Can you work these out from the model? Positions are in its coordinate system, mm. A direction names the side the tool comes from. Round coordinates to 2 decimals unless told otherwise and drop trailing zeros. Order: outer loops, then holes, each group sorted by start corner. A loop starts at its lowest first (then second) coordinate and runs counter-clockwise, first axis right, second up.
from build123d import *

# Parameters (mm, degrees)
SKETCH1_W             = 180
SKETCH1_H             = 75
BOSS_EXTRUDE1_DEPTH   = 3
SKETCH2_W             = 180
SKETCH2_H             = 4
BOSS_EXTRUDE2_DEPTH   = 17
SKETCH3_R             = 1.5
BOSS_EXTRUDE3_DEPTH   = 3
SKETCH4_R             = 0.6
CUT_EXTRUDE1_DEPTH    = 5
SKETCH5_W             = 50
SKETCH5_H             = 33
CUT_EXTRUDE2_DEPTH    = 5
F_3_0MM_DOWEL_HOLE1_D = 3
CUT_EXTRUDE3_REACH    = 100.971
SKETCH8_R             = 1.5
CUT_EXTRUDE4_REACH    = 118.366
SKETCH9_R             = 2.5


with BuildPart() as part:
    # Sketch1 → Boss-Extrude1 (new body)
    with BuildSketch(Plane(origin=(0, 0, 0), x_dir=(1, 0, 0), z_dir=(0, 1, 0))):
        Rectangle(SKETCH1_W, SKETCH1_H)
    extrude(amount=BOSS_EXTRUDE1_DEPTH)

    # Sketch2 → Boss-Extrude2 (add)
    with BuildSketch(Plane(origin=(0, 3, 0), x_dir=(1, 0, 0), z_dir=(0, 1, 0))):
        with Locations((0, 35.5)):
            Rectangle(SKETCH2_W, SKETCH2_H)
    extrude(amount=BOSS_EXTRUDE2_DEPTH)

    # Sketch3 → Boss-Extrude3 (add)
    with BuildSketch(Plane(origin=(0, 3, 0), x_dir=(1, 0, 0), z_dir=(0, 1, 0))):
        with Locations(Location((-80, 29.5, 0), (0, 0, 270))):
            Circle(SKETCH3_R)
        with Locations(Location((-55, 29.5, 0), (0, 0, 270))):
            Circle(SKETCH3_R)
        with Locations(Location((-55, -35.5, 0), (0, 0, 270))):
            Circle(SKETCH3_R)
        with Locations(Location((-80, -35.5, 0), (0, 0, 270))):
            Circle(SKETCH3_R)
    extrude(amount=BOSS_EXTRUDE3_DEPTH)

    # Sketch4 → Cut-Extrude1 (cut)
    with BuildSketch(Plane(origin=(0, 6, 0), x_dir=(1, 0, 0), z_dir=(0, 1, 0))):
        with Locations(Location((-80, 29.5, 0), (0, 0, 270))):
            Circle(SKETCH4_R)
        with Locations(Location((-55, 29.5, 0), (0, 0, 270))):
            Circle(SKETCH4_R)
        with Locations(Location((-55, -35.5, 0), (0, 0, 270))):
            Circle(SKETCH4_R)
        with Locations(Location((-80, -35.5, 0), (0, 0, 270))):
            Circle(SKETCH4_R)
    extrude(amount=-CUT_EXTRUDE1_DEPTH, mode=Mode.SUBTRACT)

    # Sketch5 → Cut-Extrude2 (cut)
    with BuildSketch(Plane(origin=(0, 3, 0), x_dir=(1, 0, 0), z_dir=(0, 1, 0))):
        with Locations((-10, -2)):
            Rectangle(SKETCH5_W, SKETCH5_H)
    extrude(amount=-CUT_EXTRUDE2_DEPTH, mode=Mode.SUBTRACT)

    # Ø3.0mm Dowel Hole1 (through all)
    with Locations(Plane(origin=(-30, 3, -18), x_dir=(0, 0, 1), z_dir=(0, 1, 0))):
        with Locations((0, 0), (0, 40), (40, 40), (40, 0)):
            Hole(F_3_0MM_DOWEL_HOLE1_D / 2)

    # Sketch8 → Cut-Extrude3 (cut, up to next)
    with BuildSketch(Plane(origin=(0, 3, 0), x_dir=(1, 0, 0), z_dir=(0, 1, 0)), mode=Mode.PRIVATE) as cut_extrude3_sk1:
        with Locations(Location((76, 22.15, 0), (0, 0, 270))):
            Circle(SKETCH8_R)
    cut_extrude3_tool1 = extrude(cut_extrude3_sk1.sketch, amount=-CUT_EXTRUDE3_REACH, mode=Mode.PRIVATE) & part.part
    # Sketch8 → Cut-Extrude3 (cut, up to next)
    with BuildSketch(Plane(origin=(0, 3, 0), x_dir=(1, 0, 0), z_dir=(0, 1, 0)), mode=Mode.PRIVATE) as cut_extrude3_sk2:
        with Locations(Location((74.7, -26.05, 0), (0, 0, 270))):
            Circle(SKETCH8_R)
    cut_extrude3_tool2 = extrude(cut_extrude3_sk2.sketch, amount=-CUT_EXTRUDE3_REACH, mode=Mode.PRIVATE) & part.part
    # Sketch8 → Cut-Extrude3 (cut, up to next)
    with BuildSketch(Plane(origin=(0, 3, 0), x_dir=(1, 0, 0), z_dir=(0, 1, 0)), mode=Mode.PRIVATE) as cut_extrude3_sk3:
        with Locations(Location((27.000808713, -10.85, 0), (0, 0, 270))):
            Circle(SKETCH8_R)
    cut_extrude3_tool3 = extrude(cut_extrude3_sk3.sketch, amount=-CUT_EXTRUDE3_REACH, mode=Mode.PRIVATE) & part.part
    # Sketch8 → Cut-Extrude3 (cut, up to next)
    with BuildSketch(Plane(origin=(0, 3, 0), x_dir=(1, 0, 0), z_dir=(0, 1, 0)), mode=Mode.PRIVATE) as cut_extrude3_sk4:
        with Locations(Location((27.000808713, 17.05, 0), (0, 0, 270))):
            Circle(SKETCH8_R)
    cut_extrude3_tool4 = extrude(cut_extrude3_sk4.sketch, amount=-CUT_EXTRUDE3_REACH, mode=Mode.PRIVATE) & part.part
    add(cut_extrude3_tool1.solids().sort_by_distance((76, 3, -22.15))[0], mode=Mode.SUBTRACT)
    add(cut_extrude3_tool2.solids().sort_by_distance((74.7, 3, 26.05))[0], mode=Mode.SUBTRACT)
    add(cut_extrude3_tool3.solids().sort_by_distance((27.000809, 3, 10.85))[0], mode=Mode.SUBTRACT)
    add(cut_extrude3_tool4.solids().sort_by_distance((27.000809, 3, -17.05))[0], mode=Mode.SUBTRACT)

    # Sketch9 → Cut-Extrude4 (cut, up to next)
    with BuildSketch(Plane.XY.offset(-33.5), mode=Mode.PRIVATE) as cut_extrude4_sk1:
        with Locations((-80, 10)):
            Circle(SKETCH9_R)
    cut_extrude4_tool1 = extrude(cut_extrude4_sk1.sketch, amount=-CUT_EXTRUDE4_REACH, mode=Mode.PRIVATE) & part.part
    # Sketch9 → Cut-Extrude4 (cut, up to next)
    with BuildSketch(Plane.XY.offset(-33.5), mode=Mode.PRIVATE) as cut_extrude4_sk2:
        with Locations((80, 10)):
            Circle(SKETCH9_R)
    cut_extrude4_tool2 = extrude(cut_extrude4_sk2.sketch, amount=-CUT_EXTRUDE4_REACH, mode=Mode.PRIVATE) & part.part
    add(cut_extrude4_tool1.solids().sort_by_distance((-80, 10, -33.5))[0], mode=Mode.SUBTRACT)
    add(cut_extrude4_tool2.solids().sort_by_distance((80, 10, -33.5))[0], mode=Mode.SUBTRACT)


solid = part.part
(1) I want a section at A-A, the plane z = -4. List the corners of the cut face in (x, y) for me, plus the area to 3 significant figures.
(2) I want a section at B-B, the plane x = -40. List the corners of the cut face in (y, z) for me.
(3) I want a section at D-D, the plane y = 17.5. List the corners of the cut face in (x, z) for me.
(4) If we mould it in two halves opening along Y, with no side actions, what happens to faces 1 (the face through (10.07, 1.48, -16.5)), 2 (the face through (-82, 8.5, -35.5)), 3 (the face through (-1, 20, -36))? For each: pulls with the +Y half, pulls with the -Y half, needs draft (parallel to the pull), parting line crosses it, or undercut.
(5) I'm going to push flat-ended pins straight in: pin 1 Ø1.8 at (x, z) = (10, -18) entering from -Y; pin 2 Ø1.3 at (x, z) = (-55, 35.5) entering from +Y; pin 3 Ø1.5 at (x, y) = (-15.5, 6.5) entering from +Z; pin 4 Ø1.5 at (x, z) = (-53.5, 19) entering from -Y. Where does each tip first touch, or does it pass through?
(6) I want a section at C-C, the plane z = -26. List the corners of the cut face in (x, y) for me, plus the area to 3 significant figures.
(7) On a 3-axis mill with a long thin cutter (end or side, diameter ignored), from which of +Z, -Z, +X, -X, +Y, -Y can I reach the whole of each face in a straight line? I mean faces 4 (the face through (-81, 6, 35)), 5 (the face through (-55, 4, -31)), 6 (the face through (-35, 2, 2)), 7 (the face through (78, 8.5, -35.5)), 8 (the face through (-1, 0, -17)). Say none if no direction works.
(8) Please list where these lines run through material, in increasing order: probe 1 along X at (y, z) = (1.85, 22); probe 2 along X at (y, z) = (2.8, -29.5); probe 3 along Y at (x, z) = (80, -35).
Ans:
1. outline: (-90, 0) - (-35, 0) - (-35, 3) - (-90, 3) - close; (15, 0) - (90, 0) - (90, 3) - (15, 3) - close
1. area: 390 mm2
2. outline: (0, -37.5) - (20, -37.5) - (20, -33.5) - (3, -33.5) - (3, 37.5) - (0, 37.5) - close
3. outline: (-90, -37.5) - (90, -37.5) - (90, -33.5) - (-90, -33.5) - close
4. face 1: needs draft
4. face 2: undercut
4. face 3: pulls with the +Y half
5. pin 1: passes through
5. pin 2: stops at y = 6
5. pin 3: stops at z = -33.5
5. pin 4: stops at y = 0
6. outline: (-90, 0) - (90, 0) - (90, 3) - (-90, 3) - close
6. area: 540 mm2
7. face 4: +Z, +X, -X, +Y
7. face 5: +Y
7. face 6: +Y, -Y
7. face 7: +Z, -Z
7. face 8: +Z, -Z, +X, -X, -Y
8. probe 1: x = -90 to -31.5, -28.5 to 8.5, 11.5 to 90
8. probe 2: x = -90 to -80.6, -79.4 to -55.6, -54.4 to 90
8. probe 3: y = 0 to 7.5, 12.5 to 20
